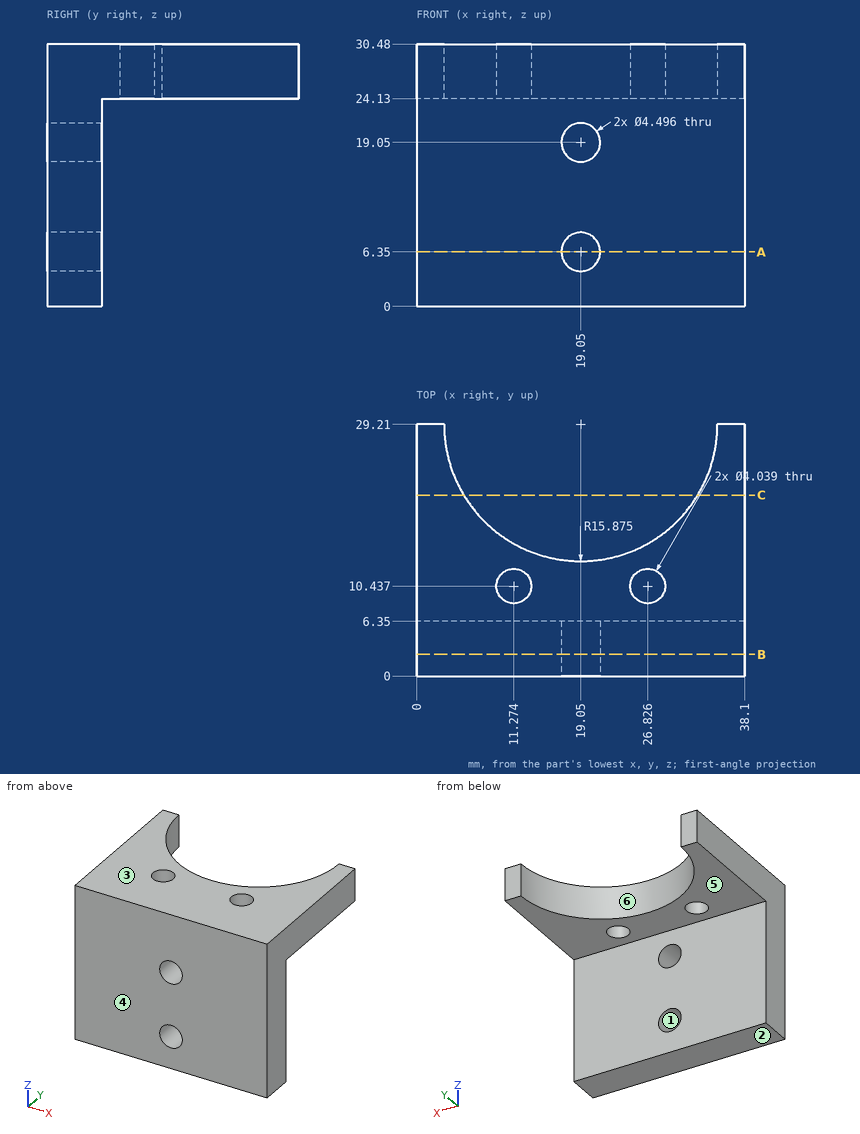
Answer from the drawing. Dimensions are ordinates in mm from the lowest x, y and z of the part. A direction names the side the tool comes from. Give positions to 0.01 mm unless a question says otherwise; leave off trailing zeros. Loops run counter-clockwise (first coordinate to the right, second up) from the corner with the lowest first, then second, coordinate; pieces in that order, holes last.
Item 1: A tool of negligible diameter and unlimited length cuts with its end or side. For the marked faces 5 and 6, from which of +Z, -Z, +X, -X, +Y, -Y can it reach the whole face along a straight path? Write none if from no direction.
Derived:
face 5: -Z, +X, -X, +Y
face 6: +Z, -Z, +Y
Item 2: Determine the mould class of the marked faces 1, 2, 3 and 4 for opening direction Z: +Z half, -Z half, draft (parallel to the pull), parting line (faces both ways), or undercut.
Derived:
face 1: undercut
face 2: -Z half
face 3: +Z half
face 4: draft
Item 3: A cutting plane is placed at B-B (y = 2.5). Give the number of separate pieces and of enclosed holes in the cut face, then the cut area to 3 significant figures.
Derived:
separate pieces: 1
enclosed holes: 2
area: 1,130 mm2
Item 4: Find the intervals of material crossed by line 1 along X through (y, z) = (2.75, 19.05); line 2 along Z through (x, y) = (4, 17); line 3 along Y through (x, z) = (10, 17), in increasing order.
Derived:
line 1: x = 0 to 16.8, 21.3 to 38.1
line 2: z = 24.13 to 30.48
line 3: y = 0 to 6.35
Item 5: A cutting plane is placed at A-A (z = 6.35). Give the vertices of the cut face in (x, y), then the cut area to 3 significant figures.
Derived:
outline: (0, 0) - (16.8, 0) - (16.8, 6.35) - (0, 6.35) - close; (21.3, 0) - (38.1, 0) - (38.1, 6.35) - (21.3, 6.35) - close
area: 213 mm2
Item 6: A cutting plane is placed at C-C (y = 21). Give the vertices of the cut face in (x, z).
Derived:
outline: (0, 24.13) - (5.46, 24.13) - (5.46, 30.48) - (0, 30.48) - close; (32.64, 24.13) - (38.1, 24.13) - (38.1, 30.48) - (32.64, 30.48) - close
Item 7: Each of these flat-tipped pins is pushed along its axis until it touches: pin 1 Ø3 at (y, z) = (8.5, 3.5) entering from -X; pin 2 Ø5.5 at (x, y) = (11.27, 10.44) entering from -Z; pin 3 Ø12 at (x, z) = (13.5, 16) entering from +Y. Where does it stop, or does it pass through?
Derived:
pin 1: passes through
pin 2: stops at z = 24.13
pin 3: stops at y = 6.35
